Read the model definition and answer for the solid it produces. Units are mm, in the model's axes. A direction names the side the tool comes from. Coordinates: 2 decimals unless noted, no trailing zeros. Loops run counter-clockwise (first coordinate to the right, second up) from the corner with the lowest first, then second, coordinate; pieces in that order, holes last. Notation, with made-up numbers: M -30.5,37.5 L -24.5,37.5 A26 cw -24.5,61.5 Z; hole C 82,-11.75 d6. An arc over 180 degrees is marked long. One line per item, written item: value. Start each with the question number.
1. Consider probe 1 along Y at (x, z) = (30, 4.5); probe 2 along X at (y, z) = (-20, 5.25) (3 decimals); probe 3 along Y at (x, z) = (0, 4). Determine where each line is inside the solid, lowest interval first.
2. The part is cut by section D-D (x = -10). Write down the section's boundary in (y, z), then the cut area to 3 significant figures.
3. The part is cut by section C-C (z = 7.75). State how many separate pieces and enclosed holes the cut face has, then the cut area to 3 significant figures.
4. The part is cut by section B-B (x = 30). Write down the section's boundary in (y, z), then the cut area to 3 significant figures.
5. A flat-ended cylindrical pin translates along its axis: pin 1 (1 mm diameter, centred on x = -8.5, y = -4.5, fed in from -Z). Find the tip coordinate at first contact, or state that the pin passes through.
6. For faces 1 (the face through (0, 14.95, 1)), 2 (the face through (37.251, 37.334, 5.07)), determine the directions among +Z, -Z, +X, -X, +Y, -Y from which every point of the face is accessible in a straight line to the end or side of a thin tool.
7. Determine the mould class of faces 3 (the face through (-1, -8, 10)), 4 (the face through (-37.329, 37.256, 5.07)), 5 (the face through (-32.024, -31.551, 4.93)) for opening direction Y: +Y half, -Y half, draft (parallel to the pull), parting line (faces both ways), or undercut.
8. The part is cut by section A-A (x = -20). Write down the section's boundary in (y, z), then the cut area to 3 significant figures.
```python
from build123d import *

# Parameters (mm, degrees)
F0_W     = 77.51
F0_H     = 77.519
F0_R     = 2.55
F0_W_2   = 29.902
F0_H_2   = 29.9
F0_R_2   = 5
F1_DEPTH = 10
F2_DEPTH = 3
F3_R     = 5


with BuildPart() as f1:
    # F0 (on Top) → F1 (new body)
    with BuildSketch(Plane.XY):
        Rectangle(F0_W, F0_H)
        with Locations((-30, -29.9995)):
            Circle(F0_R, mode=Mode.SUBTRACT)
        with Locations((-20, -19.9995)):
            Circle(F0_R, mode=Mode.SUBTRACT)
        with Locations((-10, -29.9995)):
            Circle(F0_R, mode=Mode.SUBTRACT)
        with Locations((10, -29.751634)):
            Circle(F0_R, mode=Mode.SUBTRACT)
        with Locations((0, -19.9995)):
            Circle(F0_R, mode=Mode.SUBTRACT)
        with Locations((30, -29.9995)):
            Circle(F0_R, mode=Mode.SUBTRACT)
        with Locations((20, -19.9995)):
            Circle(F0_R, mode=Mode.SUBTRACT)
        with Locations((-30, 0)):
            Circle(F0_R, mode=Mode.SUBTRACT)
        with Locations((-20, 19.9995)):
            Circle(F0_R, mode=Mode.SUBTRACT)
        with Locations((-30, 29.9995)):
            Circle(F0_R, mode=Mode.SUBTRACT)
        with Locations((-10, 29.9995)):
            Circle(F0_R, mode=Mode.SUBTRACT)
        Rectangle(F0_W_2, F0_H_2, mode=Mode.SUBTRACT)
        with Locations((30, 0)):
            Circle(F0_R, mode=Mode.SUBTRACT)
        with Locations((0, 19.9995)):
            Circle(F0_R, mode=Mode.SUBTRACT)
        with Locations((10, 29.9995)):
            Circle(F0_R, mode=Mode.SUBTRACT)
        with Locations((20, 19.9995)):
            Circle(F0_R, mode=Mode.SUBTRACT)
        with Locations((30, 29.9995)):
            Circle(F0_R, mode=Mode.SUBTRACT)
        Rectangle(F0_W_2, F0_H_2)
        Circle(F0_R_2, mode=Mode.SUBTRACT)
    extrude(amount=F1_DEPTH)

    # F0 (on Top) → F2 (cut)
    with BuildSketch(Plane.XY):
        Rectangle(F0_W_2, F0_H_2)
        Circle(F0_R_2, mode=Mode.SUBTRACT)
    extrude(amount=F2_DEPTH, mode=Mode.SUBTRACT)

    # F3
    f3_edges = [f1.edges().sort_by_distance(p)[0] for p in [
        (38.755, -38.7595, 5),
        (-38.755, -38.7595, 5),
        (38.755, 38.7595, 5),
        (-38.755, 38.7595, 5),
    ]]
    fillet(f3_edges, radius=F3_R)


solid = f1.part
```
Answer block:
1. probe 1: y = -38.76 to -32.55, -27.45 to -2.55, 2.55 to 27.45, 32.55 to 38.76
1. probe 2: x = -38.755 to -22.55, -17.45 to -2.55, 2.55 to 17.45, 22.55 to 38.755
1. probe 3: y = -38.76 to -22.55, -17.45 to -5, 5 to 17.45, 22.55 to 38.76
2. outline: M -38.76,0 L -32.55,0 L -32.55,10 L -38.76,10 Z; M -27.45,0 L -14.95,0 L -14.95,3 L 14.95,3 L 14.95,0 L 27.45,0 L 27.45,10 L -27.45,10 Z; M 32.55,0 L 38.76,0 L 38.76,10 L 32.55,10 Z
2. area: 583 mm2
3. separate pieces: 1
3. enclosed holes: 17
3. area: 5,580 mm2
4. outline: M -38.76,0 L -32.55,0 L -32.55,10 L -38.76,10 Z; M -27.45,0 L -2.55,0 L -2.55,10 L -27.45,10 Z; M 2.55,0 L 27.45,0 L 27.45,10 L 2.55,10 Z; M 32.55,0 L 38.76,0 L 38.76,10 L 32.55,10 Z
4. area: 622 mm2
5. pin 1: stops at z = 3
6. face 1: -Z
6. face 2: +Z, -Z, +X, +Y
7. face 3: draft
7. face 4: +Y half
7. face 5: undercut
8. outline: M -38.76,0 L -22.55,0 L -22.55,10 L -38.76,10 Z; M -17.45,0 L 17.45,0 L 17.45,10 L -17.45,10 Z; M 22.55,0 L 38.76,0 L 38.76,10 L 22.55,10 Z
8. area: 673 mm2
